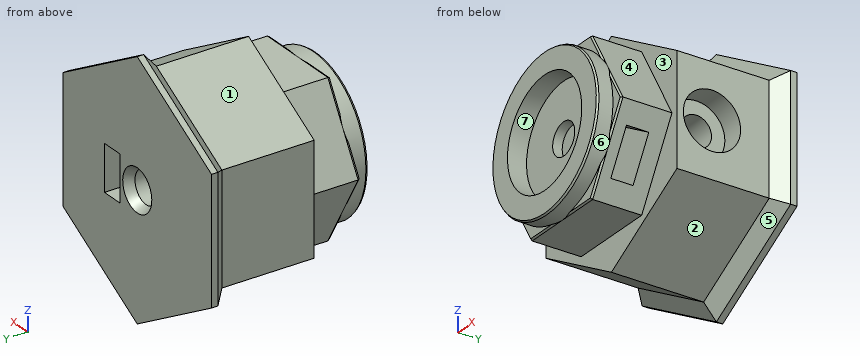
from build123d import *

# Parameters (mm, degrees)
SKIZZE1_R                       = 2.525
AUFSATZ_LINEAR_AUSTRAGEN1_DEPTH = 28
SKIZZE2_W                       = 3.5
SKIZZE2_H                       = 7.2
SCHNITT_LINEAR_AUSTRAGEN1_DEPTH = 16.2
SKIZZE4_R                       = 2.4
SCHNITT_LINEAR_AUSTRAGEN2_DEPTH = 16
SKIZZE6_R                       = 14.009035946
AUFSATZ_LINEAR_AUSTRAGEN3_DEPTH = 3
SKIZZE7_R                       = 20
SCHNITT_LINEAR_AUSTRAGEN4_DEPTH = 10.5
FASE1_SIZE                      = 0.8
FASE1_SIZE2                     = 1.385640646
SKIZZE9_W                       = 7.2
SKIZZE9_H                       = 3.5
SCHNITT_LINEAR_AUSTRAGEN5_DEPTH = 16
SKIZZE10_R                      = 8.5
SCHNITT_LINEAR_AUSTRAGEN6_DEPTH = 3
FASE2_SIZE                      = 2
SKIZZE11_R                      = 4.5
SCHNITT_LINEAR_AUSTRAGEN7_DEPTH = 3.6
SKIZZE12_R                      = 14.338361474
SKIZZE12_R_2                    = 12
SCHNITT_LINEAR_AUSTRAGEN8_DEPTH = 2.5
FASE3_SIZE                      = 0.3
FASE3_SIZE2                     = 0.173205081
FASE4_SIZE                      = 0.173205081
FASE4_SIZE_2                    = 0.3


# Some blends are built 0.0001 mm under size
with BuildPart() as part:
    # Skizze1 → Aufsatz-Linear austragen1 (new body)
    with BuildSketch(Plane(origin=(0, 0, 0), x_dir=(1, 0, 0), z_dir=(0, 1, 0))):
        Polygon((15, 8.660254038), (0, 17.320508076), (-15, 8.660254038), (-15, -8.660254038), (0, -17.320508076), (15, -8.660254038), align=None)
        with Locations(Location((0, 0, 0), (0, 0, 270))):
            Circle(SKIZZE1_R, mode=Mode.SUBTRACT)
    extrude(amount=AUFSATZ_LINEAR_AUSTRAGEN1_DEPTH)

    # Skizze2 → Schnitt-Linear austragen1 (cut)
    with BuildSketch(Plane(origin=(0, 28, 0), x_dir=(1, 0, 0), z_dir=(0, 1, 0))):
        with Locations((5.75, 0)):
            Rectangle(SKIZZE2_W, SKIZZE2_H)
    extrude(amount=-SCHNITT_LINEAR_AUSTRAGEN1_DEPTH, mode=Mode.SUBTRACT)

    # Skizze4 → Schnitt-Linear austragen2 (cut)
    with BuildSketch(Plane(origin=(15, 0, 0), x_dir=(0, 0, -1), z_dir=(1, 0, 0))):
        with Locations((0, 16)):
            Circle(SKIZZE4_R)
    extrude(amount=-SCHNITT_LINEAR_AUSTRAGEN2_DEPTH, mode=Mode.SUBTRACT)

    # Skizze6 → Aufsatz-Linear austragen3 (add)
    with BuildSketch(Plane(origin=(0, 28, 0), x_dir=(1, 0, 0), z_dir=(0, 1, 0))):
        Polygon((0, -19.629909152), (17, -9.814954576), (17, 9.814954576), (0, 19.629909152), (-17, 9.814954576), (-17, -9.814954576), align=None)
        Circle(SKIZZE6_R, mode=Mode.SUBTRACT)
    extrude(amount=-AUFSATZ_LINEAR_AUSTRAGEN3_DEPTH)

    # Skizze7 → Schnitt-Linear austragen4 (cut)
    with BuildSketch(Plane.XZ):
        Circle(SKIZZE7_R)
        Polygon((-6.92820323, 12), (-13.856406461, 0), (-6.92820323, -12), (6.92820323, -12), (13.856406461, 0), (6.92820323, 12), align=None, mode=Mode.SUBTRACT)
    extrude(amount=-SCHNITT_LINEAR_AUSTRAGEN4_DEPTH, mode=Mode.SUBTRACT)

    # Fase1
    fase1_edges = [part.edges().sort_by_distance(p)[0] for p in [
        (0, 28, -2.525),
    ]]
    fase1_side = [part.faces().sort_by_distance(p)[0] for p in [
        (0, 28, -3.044358579),
    ]]
    chamfer(fase1_edges, length=FASE1_SIZE, length2=FASE1_SIZE2, reference=fase1_side[0])

    # Skizze9 → Schnitt-Linear austragen5 (cut)
    with BuildSketch(Plane(origin=(10.392304845, 0, -6), x_dir=(-0.49999999999999983, 0, -0.8660254037844387), z_dir=(0.8660254037844387, 0, -0.49999999999999983))):
        with Locations((0, 6.25)):
            Rectangle(SKIZZE9_W, SKIZZE9_H)
    extrude(amount=-SCHNITT_LINEAR_AUSTRAGEN5_DEPTH, mode=Mode.SUBTRACT)

    # Skizze10 → Schnitt-Linear austragen6 (cut)
    with BuildSketch(Plane.XZ):
        with Locations(Location((0, 0, 0), (0, 0, 270))):
            Circle(SKIZZE10_R)
    extrude(amount=-SCHNITT_LINEAR_AUSTRAGEN6_DEPTH, mode=Mode.SUBTRACT)

    # Fase2
    fase2_edges = [part.edges().sort_by_distance(p)[0] for p in [
        (-8.5, 25, 14.722431864),
        (-17, 25, 0),
        (-8.5, 25, -14.722431864),
        (8.5, 25, -14.722431864),
        (17, 25, 0),
        (8.5, 25, 14.722431864),
    ]]
    chamfer(fase2_edges, length=FASE2_SIZE - 0.0001)  # a hair under: the kernel refuses the full size

    # Skizze11 → Schnitt-Linear austragen7 (cut)
    with BuildSketch(Plane(origin=(15, 0, 0), x_dir=(0, 0, -1), z_dir=(1, 0, 0))):
        with Locations((0, 16)):
            Circle(SKIZZE11_R)
    extrude(amount=-SCHNITT_LINEAR_AUSTRAGEN7_DEPTH, mode=Mode.SUBTRACT)

    # Skizze12 → Schnitt-Linear austragen8 (cut)
    with BuildSketch(Plane.XZ):
        Circle(SKIZZE12_R)
        with Locations(Location((0, 0, 0), (0, 0, 270))):
            Circle(SKIZZE12_R_2, mode=Mode.SUBTRACT)
    extrude(amount=-SCHNITT_LINEAR_AUSTRAGEN8_DEPTH, mode=Mode.SUBTRACT)

    # Fase3
    fase3_edges = [part.edges().sort_by_distance(p)[0] for p in [
        (0, 0, 12),
    ]]
    fase3_side = [part.faces().sort_by_distance(p)[0] for p in [
        (0, 1.25, 12),
    ]]
    chamfer(fase3_edges, length=FASE3_SIZE, length2=FASE3_SIZE2, reference=fase3_side[0])

    # Fase4
    # the kernel refuses this chamfer: 0.3, 0.173205081 mm, written as the material it takes off along each edge
    with BuildSketch(Plane(origin=(-10.392304845, 2.5, 6), x_dir=(0.864572857266567, -0.05789386240267096, -0.4991613718768963), z_dir=(0.5, 0, 0.8660254037844387))) as fase4_piece_1_section:
        Polygon((FASE4_SIZE * 0.998322742353, FASE4_SIZE * 0.0578938623214), (-FASE4_SIZE_2 * 0.0578938624027, FASE4_SIZE_2 * 0.998322743754), (0, 0), align=None)
    fase4_piece_1 = extrude(amount=7.704328957, mode=Mode.PRIVATE)
    fase4_piece_1 = fase4_piece_1 - Plane(origin=(0, 2.602492353, 0), x_dir=(0, 0, -1), z_dir=(0, -1, 0)) * Cylinder(12, 17, mode=Mode.PRIVATE)
    add(fase4_piece_1, mode=Mode.SUBTRACT)
    with BuildSketch(Plane(origin=(-14.244469324, 2.5, -0.672144596), x_dir=(0.864572857266567, -0.05789386240267102, -0.4991613718768963), z_dir=(0.5, 0, 0.8660254037844387))) as fase4_piece_2_section:
        Polygon((FASE4_SIZE * 0.998322742353, FASE4_SIZE * 0.0578938623214), (-FASE4_SIZE_2 * 0.0578938624027, FASE4_SIZE_2 * 0.998322743754), (0, 0), align=None)
    fase4_piece_2 = extrude(amount=7.704328957, mode=Mode.PRIVATE)
    fase4_piece_2 = fase4_piece_2 - Plane(origin=(0, 2.602492354, 0), x_dir=(0, 0, -1), z_dir=(0, -1, 0)) * Cylinder(12, 17, mode=Mode.PRIVATE)
    add(fase4_piece_2, mode=Mode.SUBTRACT)
    with BuildSketch(Plane(origin=(-7.704328957, 2.5, 12), x_dir=(0, -0.057893862402670936, -0.9983227437537926), z_dir=(1, 0, 0))) as fase4_piece_3_section:
        Polygon((FASE4_SIZE * 0.998322742353, FASE4_SIZE * 0.0578938623214), (-FASE4_SIZE_2 * 0.0578938624027, FASE4_SIZE_2 * 0.998322743754), (0, 0), align=None)
    fase4_piece_3 = extrude(amount=7.704328957, mode=Mode.PRIVATE)
    fase4_piece_3 = fase4_piece_3 - Plane(origin=(0, 2.602492354, 0), x_dir=(0, 0, -1), z_dir=(0, -1, 0)) * Cylinder(12, 17, mode=Mode.PRIVATE)
    add(fase4_piece_3, mode=Mode.SUBTRACT)
    with BuildSketch(Plane(origin=(0, 2.5, 12), x_dir=(0, -0.057893862402670936, -0.9983227437537926), z_dir=(1, 0, 0))) as fase4_piece_4_section:
        Polygon((FASE4_SIZE * 0.998322742353, FASE4_SIZE * 0.0578938623214), (-FASE4_SIZE_2 * 0.0578938624027, FASE4_SIZE_2 * 0.998322743754), (0, 0), align=None)
    fase4_piece_4 = extrude(amount=7.704328957, mode=Mode.PRIVATE)
    fase4_piece_4 = fase4_piece_4 - Plane(origin=(0, 2.602492353, 0), x_dir=(0, 0, -1), z_dir=(0, -1, 0)) * Cylinder(12, 17, mode=Mode.PRIVATE)
    add(fase4_piece_4, mode=Mode.SUBTRACT)
    with BuildSketch(Plane(origin=(6.540140367, 2.5, 12.672144596), x_dir=(-0.864572857266567, -0.05789386240267135, -0.49916137187689613), z_dir=(0.4999999999999999, 0, -0.8660254037844388))) as fase4_piece_5_section:
        Polygon((FASE4_SIZE * 0.998322742353, FASE4_SIZE * 0.0578938623214), (-FASE4_SIZE_2 * 0.0578938624027, FASE4_SIZE_2 * 0.998322743754), (0, 0), align=None)
    fase4_piece_5 = extrude(amount=7.704328957, mode=Mode.PRIVATE)
    fase4_piece_5 = fase4_piece_5 - Plane(origin=(0, 2.602492354, 0), x_dir=(0, 0, -1), z_dir=(0, -1, 0)) * Cylinder(12, 17, mode=Mode.PRIVATE)
    add(fase4_piece_5, mode=Mode.SUBTRACT)
    with BuildSketch(Plane(origin=(10.392304845, 2.5, 6), x_dir=(-0.864572857266567, -0.05789386240267096, -0.49916137187689613), z_dir=(0.4999999999999999, 0, -0.8660254037844388))) as fase4_piece_6_section:
        Polygon((FASE4_SIZE * 0.998322742353, FASE4_SIZE * 0.0578938623214), (-FASE4_SIZE_2 * 0.0578938624027, FASE4_SIZE_2 * 0.998322743754), (0, 0), align=None)
    fase4_piece_6 = extrude(amount=7.704328957, mode=Mode.PRIVATE)
    fase4_piece_6 = fase4_piece_6 - Plane(origin=(0, 2.602492353, 0), x_dir=(0, 0, -1), z_dir=(0, -1, 0)) * Cylinder(12, 17, mode=Mode.PRIVATE)
    add(fase4_piece_6, mode=Mode.SUBTRACT)
    with BuildSketch(Plane(origin=(14.244469324, 2.5, 0.672144596), x_dir=(-0.8645728572665671, -0.05789386240267102, 0.49916137187689597), z_dir=(-0.49999999999999967, 0, -0.8660254037844388))) as fase4_piece_7_section:
        Polygon((FASE4_SIZE * 0.998322742353, FASE4_SIZE * 0.0578938623214), (-FASE4_SIZE_2 * 0.0578938624027, FASE4_SIZE_2 * 0.998322743754), (0, 0), align=None)
    fase4_piece_7 = extrude(amount=7.704328957, mode=Mode.PRIVATE)
    fase4_piece_7 = fase4_piece_7 - Plane(origin=(0, 2.602492354, 0), x_dir=(0, 0, -1), z_dir=(0, -1, 0)) * Cylinder(12, 17, mode=Mode.PRIVATE)
    add(fase4_piece_7, mode=Mode.SUBTRACT)
    with BuildSketch(Plane(origin=(10.392304845, 2.5, -6), x_dir=(-0.8645728572665671, -0.05789386240267096, 0.499161371876896), z_dir=(-0.49999999999999967, 0, -0.8660254037844388))) as fase4_piece_8_section:
        Polygon((FASE4_SIZE * 0.998322742353, FASE4_SIZE * 0.0578938623214), (-FASE4_SIZE_2 * 0.0578938624027, FASE4_SIZE_2 * 0.998322743754), (0, 0), align=None)
    fase4_piece_8 = extrude(amount=7.704328957, mode=Mode.PRIVATE)
    fase4_piece_8 = fase4_piece_8 - Plane(origin=(0, 2.602492353, 0), x_dir=(0, 0, -1), z_dir=(0, -1, 0)) * Cylinder(12, 17, mode=Mode.PRIVATE)
    add(fase4_piece_8, mode=Mode.SUBTRACT)
    with BuildSketch(Plane(origin=(7.704328957, 2.5, -12), x_dir=(0, -0.057893862402670936, 0.9983227437537926), z_dir=(-1, 0, 0))) as fase4_piece_9_section:
        Polygon((FASE4_SIZE * 0.998322742353, FASE4_SIZE * 0.0578938623214), (-FASE4_SIZE_2 * 0.0578938624027, FASE4_SIZE_2 * 0.998322743754), (0, 0), align=None)
    fase4_piece_9 = extrude(amount=7.704328957, mode=Mode.PRIVATE)
    fase4_piece_9 = fase4_piece_9 - Plane(origin=(0, 2.602492354, 0), x_dir=(0, 0, -1), z_dir=(0, -1, 0)) * Cylinder(12, 17, mode=Mode.PRIVATE)
    add(fase4_piece_9, mode=Mode.SUBTRACT)
    with BuildSketch(Plane(origin=(0, 2.5, -12), x_dir=(0, -0.057893862402670936, 0.9983227437537926), z_dir=(-1, 0, 0))) as fase4_piece_10_section:
        Polygon((FASE4_SIZE * 0.998322742353, FASE4_SIZE * 0.0578938623214), (-FASE4_SIZE_2 * 0.0578938624027, FASE4_SIZE_2 * 0.998322743754), (0, 0), align=None)
    fase4_piece_10 = extrude(amount=7.704328957, mode=Mode.PRIVATE)
    fase4_piece_10 = fase4_piece_10 - Plane(origin=(0, 2.602492354, 0), x_dir=(0, 0, -1), z_dir=(0, -1, 0)) * Cylinder(12, 17, mode=Mode.PRIVATE)
    add(fase4_piece_10, mode=Mode.SUBTRACT)
    with BuildSketch(Plane(origin=(-6.540140367, 2.5, -12.672144596), x_dir=(0.864572857266567, -0.05789386240267136, 0.49916137187689624), z_dir=(-0.4999999999999999, 0, 0.8660254037844387))) as fase4_piece_11_section:
        Polygon((FASE4_SIZE * 0.998322742353, FASE4_SIZE * 0.0578938623214), (-FASE4_SIZE_2 * 0.0578938624027, FASE4_SIZE_2 * 0.998322743754), (0, 0), align=None)
    fase4_piece_11 = extrude(amount=7.704328957, mode=Mode.PRIVATE)
    fase4_piece_11 = fase4_piece_11 - Plane(origin=(0, 2.602492354, 0), x_dir=(0, 0, -1), z_dir=(0, -1, 0)) * Cylinder(12, 17, mode=Mode.PRIVATE)
    add(fase4_piece_11, mode=Mode.SUBTRACT)
    with BuildSketch(Plane(origin=(-10.392304845, 2.5, -6), x_dir=(0.864572857266567, -0.05789386240267096, 0.49916137187689624), z_dir=(-0.4999999999999999, 0, 0.8660254037844387))) as fase4_piece_12_section:
        Polygon((FASE4_SIZE * 0.998322742353, FASE4_SIZE * 0.0578938623214), (-FASE4_SIZE_2 * 0.0578938624027, FASE4_SIZE_2 * 0.998322743754), (0, 0), align=None)
    fase4_piece_12 = extrude(amount=7.704328957, mode=Mode.PRIVATE)
    fase4_piece_12 = fase4_piece_12 - Plane(origin=(0, 2.602492353, 0), x_dir=(0, 0, -1), z_dir=(0, -1, 0)) * Cylinder(12, 17, mode=Mode.PRIVATE)
    add(fase4_piece_12, mode=Mode.SUBTRACT)


solid = part.part
Design review of the part built by this model. Coordinates are the model's own, in mm. Face numbers are marked on the shaded views. A direction names the side the tool comes from. Round coordinates to 2 decimals unless told otherwise and drop trailing zeros. One line per item, written item: value. Start each with the question number.
1) Insertion check: pin 1 Ø1.5 at (y, z) = (13, -13.5) entering from +X; pin 2 Ø2.5 at (x, y) = (1.5, 5.5) entering from +Z; pin 3 Ø1 at (x, y) = (-2, 7) entering from -Z; pin 4 Ø3 at (x, z) = (0, 0) entering from +Y. Each pin has a flat end and moves straight along its axis. Give the tip position at first contact, or say it passes through.
2) To check wall thickness, follow L1, parallel to X at y = 0.6, z = 0; L2, parallel to Z at x = 0, y = 15.25 (1 decimal); L3, parallel to Z at x = 0, y = 3.9 (3 decimals). State the ranges of each line that lie inside material, in increasing order. Write a range as from..to.
3) Draft analysis for pull direction X (two halves, no side actions). For the marked faces 5, 6 and 7, state which applies: +X half, -X half, draft (parallel to the pull), parting line (faces both ways), or undercut.
4) For the marked faces 1, 2, 3 and 4, list the 3-axis set-ups (+Z, -Z, +X, -X, +Y, -Y) from which the entire face can be reached by the end or side of a thin tool; tool diameter is ignored.
5) Consider section C-C on x = 8. Give the number of separate pieces and of enclosed holes in the cut face, then the cut area to 3 significant figures.
Reported:
1. pin 1: stops at x = 7.92
1. pin 2: stops at z = 12
1. pin 3: stops at z = -12
1. pin 4: passes through
2. L1: x = -12..-8.5, 8.5..12
2. L2: z = -17.3..-2.5, 2.5..17.3
2. L3: z = -12..-2.525, 2.525..12
3. face 5: +X half
3. face 6: parting line
3. face 7: undercut
4. face 1: +Z, -X, -Y
4. face 2: -Z, +X, -Y
4. face 3: -Y
4. face 4: +Z, +X, -Y
5. separate pieces: 1
5. enclosed holes: 2
5. area: 596 mm^2
